from build123d import *

# Parameters (mm, degrees)
SKETCH1_R           = 78.359
SKETCH1_R_2         = 76.2
BOSS_EXTRUDE1_DEPTH = 50.8
SKETCH4_R           = 6.35
CUT_EXTRUDE1_DEPTH  = 25.4
SKETCH5_R           = 6.35
CUT_EXTRUDE2_DEPTH  = 25.4
SKETCH6_R           = 2.7305
CUT_EXTRUDE3_DEPTH  = 2.54
CIRPATTERN1_COUNT   = 4
CIRPATTERN1_ANGLE   = 240


with BuildPart() as part:
    # Sketch1 → Boss-Extrude1 (new body)
    with BuildSketch(Plane(origin=(0, 0, 0), x_dir=(1, 0, 0), z_dir=(0, 1, 0))):
        with Locations(Location((0, 0, 0), (0, 0, 270))):
            Circle(SKETCH1_R)
        with Locations(Location((0, 0, 0), (0, 0, 270))):
            Circle(SKETCH1_R_2, mode=Mode.SUBTRACT)
    extrude(amount=BOSS_EXTRUDE1_DEPTH)

    # Sketch4 → Cut-Extrude1 (cut)
    with BuildSketch(Plane(origin=(33.115944372, 0, 71.017371884), x_dir=(0, -1, 0), z_dir=(0.4226182617407003, 0, 0.9063077870366496))):
        with Locations(Location((-25.4, 0, 0), (0, 0, 90))):
            Circle(SKETCH4_R)
    extrude(amount=-CUT_EXTRUDE1_DEPTH, mode=Mode.SUBTRACT)

    # Sketch5 → Cut-Extrude2 (cut)
    with BuildSketch(Plane(origin=(-33.115944372, 0, 71.017371884), x_dir=(0, -1, 0), z_dir=(-0.4226182617407003, 0, 0.9063077870366496))):
        with Locations(Location((-25.4, 0, 0), (0, 0, 90))):
            Circle(SKETCH5_R)
    extrude(amount=-CUT_EXTRUDE2_DEPTH, mode=Mode.SUBTRACT)

    # Sketch6 → Cut-Extrude3 (cut)
    with BuildSketch(Plane(origin=(67.860884615, 0, 39.1795), x_dir=(0, -1, 0), z_dir=(0.8660254037844416, 0, 0.49999999999999495))):
        with Locations(Location((-25.4, 0, 0), (0, 0, 90))):
            Circle(SKETCH6_R)
    cut_extrude3 = extrude(amount=-CUT_EXTRUDE3_DEPTH, mode=Mode.SUBTRACT)

    # CirPattern1: Cut-Extrude3 ×4 about axis
    cirpattern1_axis = Axis((0, 50.8, 0), (0, 1, 0))
    for i in range(1, CIRPATTERN1_COUNT):
        add(cut_extrude3.rotate(cirpattern1_axis, i * CIRPATTERN1_ANGLE / (CIRPATTERN1_COUNT - 1)), mode=Mode.SUBTRACT)


solid = part.part
Could you check a few things on this model? Use its own coordinates, in mm. Give positions to 0.01 mm unless a question says otherwise; leave off trailing zeros. Order: outer loops, then holes, each group sorted by start corner. A loop starts at its lowest first (then second) coordinate and runs counter-clockwise, first axis right, second up. Notation, with made-up numbers: (-20.75, -13.75) - (27.25, -13.75) arc R18 cw to (27.25, -6.75) - close; hole circle Ø9 at (59, -40). An arc over 180 degrees is marked (long way). One line per question, with ' | ' between items. Start each with the question number.
Item 1: I want a section at A-A on z = 0. Write out the boundary of the cut face in (x, y), then the cut area to 3 significant figures.
Item 2: Thinking about a two-plate mould opening in Y: for faces 1 (the cylindrical face through (50.122, 22.734, -58.812)), 2 (the flat face through (-75, 0, 17)), 3 (the flat face through (-75, 50.8, 17)), which applies, pulls with the +Y half, pulls with the -Y half, needs draft (parallel to the pull), parting line crosses it, or undercut?
Item 3: I'm going to push flat-ended pins straight in: pin 1 Ø1.5 at (y, z) = (33.5, -31.5) entering from -X; pin 2 Ø12 at (y, z) = (25, 19) entering from -X; pin 3 Ø4 at (y, z) = (30, 39.5) entering from -X. Where does each tip first touch, or does it pass through?
Item 4: I want a section at B-B on x = 0. Write out the boundary of the cut face in (y, z).
Item 5: I want a section at C-C on y = 39. Write out the boundary of the cut face in (x, z), then the cut area to 3 significant figures.
Item 6: I need wall thicknesses on probe 1 along X at (y, z) = (32.5, 0); probe 2 along Z at (x, y) = (-23.5, 45.5); probe 3 along Z at (x, y) = (-69, 27). Which ranges of each line are inside material? Lowest first, please. Write a range as [from, to].
Verdict:
1) outline: (-78.36, 0) - (-76.2, 0) - (-76.2, 50.8) - (-78.36, 50.8) - close; (76.2, 0) - (78.36, 0) - (78.36, 50.8) - (76.2, 50.8) - close | area: 219 mm^2
2) face 1: undercut | face 2: pulls with the -Y half | face 3: pulls with the +Y half
3) pin 1: x = -72.07 | pin 2: x = -77.27 | pin 3: x = -68.8
4) outline: (0, -78.36) - (50.8, -78.36) - (50.8, -76.2) - (0, -76.2) - close; (0, 76.2) - (50.8, 76.2) - (50.8, 78.36) - (0, 78.36) - close
5) outline: circle Ø156.72 at (0, 0); hole circle Ø152.4 at (0, 0) | area: 1,050 mm^2
6) probe 1: [-78.36, -76.2], [76.2, 78.36] | probe 2: [-74.75, -72.49], [72.49, 74.75] | probe 3: [-37.14, -32.33], [32.33, 37.14]
